Could you check a few things on this drawing? It's one solid part, dimensions in mm from its lowest x, y, z. A direction names the side the tool comes from. Coordinates: 2 decimals unless noted, no trailing zeros. Loops run counter-clockwise (first coordinate to the right, second up) from the corner with the lowest first, then second, coordinate; pieces in that order, holes last.
1) Imagine slicing it at D-D on z = 26. Please give me the cut outline in (x, y), plus the area to 3 significant figures.
2) Imagine slicing it at C-C on x = 1.75. Please give me the cut outline in (y, z).
3) For the marked faces 1 and 2, which set-ups out of +Z, -Z, +X, -X, +Y, -Y let a thin tool reach every point of the face, with its end or its side?
4) Imagine slicing it at A-A on z = 20. Please give me the cut outline in (x, y).
5) If I drill on line 1 along Y through (x, z) = (10, 20); line 2 along X through (y, z) = (2.5, 10.5); line 3 along Z through (x, y) = (4, 19.5), over which ranges is the centre line in solid material (lowest first)?
6) Will these pins go through, and if not, where does the flat tip stop? P1, Ø8, axis at x = 5.5, z = 25.5, coming from the +Y side; P2, Ø8, axis at x = 12.5, z = 15, coming from the -Y side (3 decimals); P3, Ø1.5, axis at x = 13, y = 31, coming from the -Z side.
7) Thinking about a two-plate mould opening in X: for the marked faces 3, 4, 5 and 6, which applies, released by +X, released by -X, zero draft, split by the parting line, or undercut?
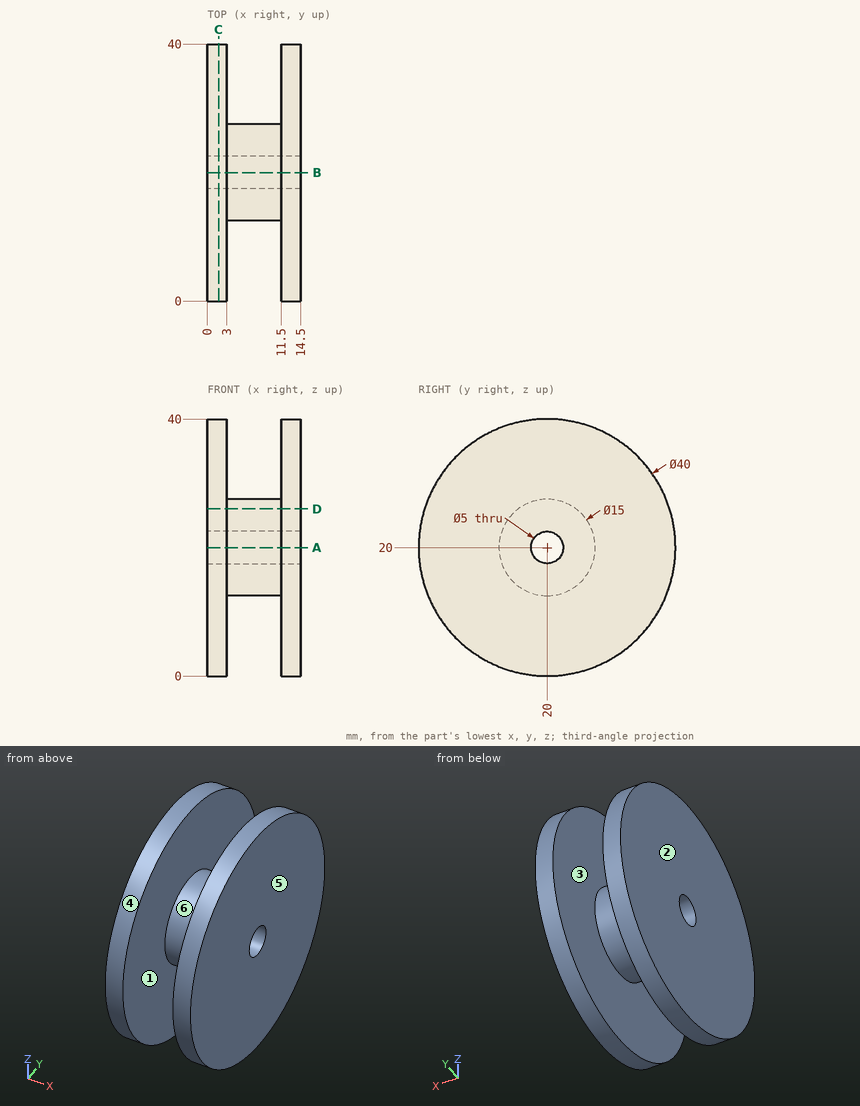
Filled in:
1. outline: (0, 0.92) - (3, 0.92) - (3, 15.5) - (11.5, 15.5) - (11.5, 0.92) - (14.5, 0.92) - (14.5, 39.08) - (11.5, 39.08) - (11.5, 24.5) - (3, 24.5) - (3, 39.08) - (0, 39.08) - close
1. area: 305 mm2
2. outline: circle Ø40 at (20, 20); hole circle Ø5 at (20, 20)
3. face 1: none
3. face 2: +Z, -Z, -X, +Y, -Y
4. outline: (0, 0) - (3, 0) - (3, 12.5) - (11.5, 12.5) - (11.5, 0) - (14.5, 0) - (14.5, 17.5) - (0, 17.5) - close; (0, 22.5) - (14.5, 22.5) - (14.5, 40) - (11.5, 40) - (11.5, 27.5) - (3, 27.5) - (3, 40) - (0, 40) - close
5. line 1: y = 12.5 to 17.5, 22.5 to 27.5
5. line 2: x = 0 to 3, 11.5 to 14.5
5. line 3: z = 12.52 to 17.55, 22.45 to 27.48
6. P1: stops at y = 39.86
6. P2: stops at y = 0.025
6. P3: stops at z = 2.83
7. face 3: undercut
7. face 4: zero draft
7. face 5: released by +X
7. face 6: undercut
